Check sheet for the modelled part. Datum: model origin and axes. Units: mm. Face numbers are marked on the shaded views. A direction names the side the tool comes from. Coordinates: 2 decimals unless noted, no trailing zeros. Write each loop counter-clockwise with the first axis right and the second up, starting at its lowest first coordinate (ties: lowest second). Pieces come first, ordered by that corner, then holes. Notation, with made-up numbers: (24.25, -39.5) - (61.25, -39.5) arc R20 cw to (61.25, -15.5) - close; hole circle Ø7 at (6, 24.25). An arc over 180 degrees is marked (long way). Write each question's results on one line, items separated by ' | '.
from build123d import *

# Parameters (mm, degrees)
PAD001_DEPTH  = 6
PAD002_DEPTH  = 8
ARRAY_COUNT   = 30
SKETCH_R      = 15
SKETCH_R_2    = 1.8
PAD_DEPTH     = 8
SKETCH003_R   = 5
SKETCH003_R_2 = 3
PAD003_DEPTH  = 1


with BuildPart() as nutmount:
    # Sketch001 → Pad001 (new body)
    with BuildSketch(Plane.XY):
        Polygon((1.6, -2.7712812921), (3.2, 0), (1.6, 2.7712812921), (-1.6, 2.7712812921), (-3.2, 0), (-1.6, -2.7712812921), align=None)
    extrude(amount=PAD001_DEPTH)


with BuildPart() as cutblock:
    # Sketch002 → Pad002 (new body)
    with BuildSketch(Plane.XY):
        with BuildLine():
            ThreePointArc((1, 14.9666295471), (0, 15), (-1, 14.9666295471))
            Line((-1, 14.9666295471), (-0.5, 13.9910685796))
            ThreePointArc((0.5, 13.9910685796), (0, 14), (-0.5, 13.9910685796))
            Line((1, 14.9666295471), (0.5, 13.9910685796))
        make_face()
    extrude(amount=PAD002_DEPTH)

    # Array: CutBlock ×30 about axis
    array_axis = Axis((0, 0, 0), (0, 0, 1))


with BuildPart() as cutblock_1:
    add(cutblock.part)
    for i in range(1, ARRAY_COUNT):
        add(cutblock.part.rotate(array_axis, i * 360 / ARRAY_COUNT))

    # Fusion001: union NutMount
    add(nutmount.part)


with BuildPart() as base:
    # Sketch → Pad (new body)
    with BuildSketch(Plane.XY):
        Circle(SKETCH_R)
        Circle(SKETCH_R_2, mode=Mode.SUBTRACT)
    extrude(amount=PAD_DEPTH)


with BuildPart() as final:
    # Sketch003 → Pad003 (new body)
    with BuildSketch(Plane.XY.offset(8)):
        Circle(SKETCH003_R)
        Circle(SKETCH003_R_2, mode=Mode.SUBTRACT)
    extrude(amount=PAD003_DEPTH)

    # Fusion: union Base
    add(base.part)

    # Cut: cut CutBlock
    add(cutblock_1.part, mode=Mode.SUBTRACT)


solid = final.part
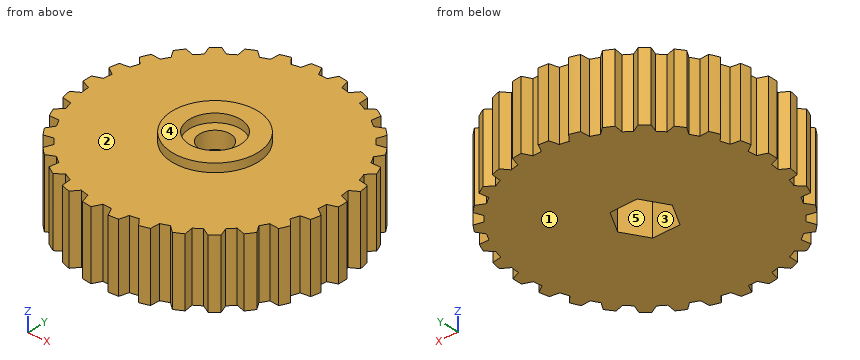
1. Material ranges on L1, parallel to X at y = 0, z = 7.25; L2, parallel to Y at x = 0, z = 8.35; L3, parallel to X at y = 13, z = 3, recorded low to high. Write a range as [from, to].
Values follow:
L1: x = [-15, -1.8], [1.8, 15] | L2: y = [-5, -3], [3, 5] | L3: x = [-7.48, -6.67], [-5.23, 5.23], [6.67, 7.48]
2. Sectioned sample at A-A (x = 0). Record the cut outline in (y, z).
Values follow:
outline: (-14, 0) - (-2.77, 0) - (-2.77, 6) - (-1.8, 6) - (-1.8, 8) - (-3, 8) - (-3, 9) - (-5, 9) - (-5, 8) - (-14, 8) - close; (1.8, 6) - (2.77, 6) - (2.77, 0) - (14, 0) - (14, 8) - (5, 8) - (5, 9) - (3, 9) - (3, 8) - (1.8, 8) - close
3. Go/stop test with flat-tipped pins: pin 1 (4 mm diameter, centred on x = 7.5, z = 8, fed in from +Y); pin 2 (5 mm diameter, centred on x = 4, z = 4.5, fed in from -Y); pin 3 (1.5 mm diameter, centred on x = -10, y = -4, fed in from +Z). Record where each tip stops, or that it passes through.
Values follow:
pin 1: stops at y = 13.27 | pin 2: stops at y = -14.92 | pin 3: stops at z = 8
4. Access from +Z, -Z, +X, -X, +Y, -Y to the whole of each face (thin tool, end or side, straight path). Record for the marked faces 1, 2 and 3.
Values follow:
face 1: -Z, +X, -X, +Y, -Y | face 2: +Z | face 3: -Z
5. Draft check along Y on the marked faces 4 and 5. Enter one of: pulls with the +Y half, pulls with the -Y half, needs draft (parallel to the pull), parting line crosses it, or undercut.
Values follow:
face 4: needs draft | face 5: undercut
